Check sheet for the drawn part. Datum: minimum x, y, z corner. Units: mm. Coordinates: 2 decimals unless noted, no trailing zeros. Order: outer loops, then holes, each group sorted by start corner. A loop starts at its lowest first (then second) coordinate and runs counter-clockwise, first axis right, second up. Notation, with made-up numbers: (-20, 10.25) - (-7, 10.25) arc R16 ccw to (-7, 14.25) - close; hole circle Ø7 at (28.5, 34.5). An arc over 180 degrees is marked (long way). Put each result on its own line as item: value.
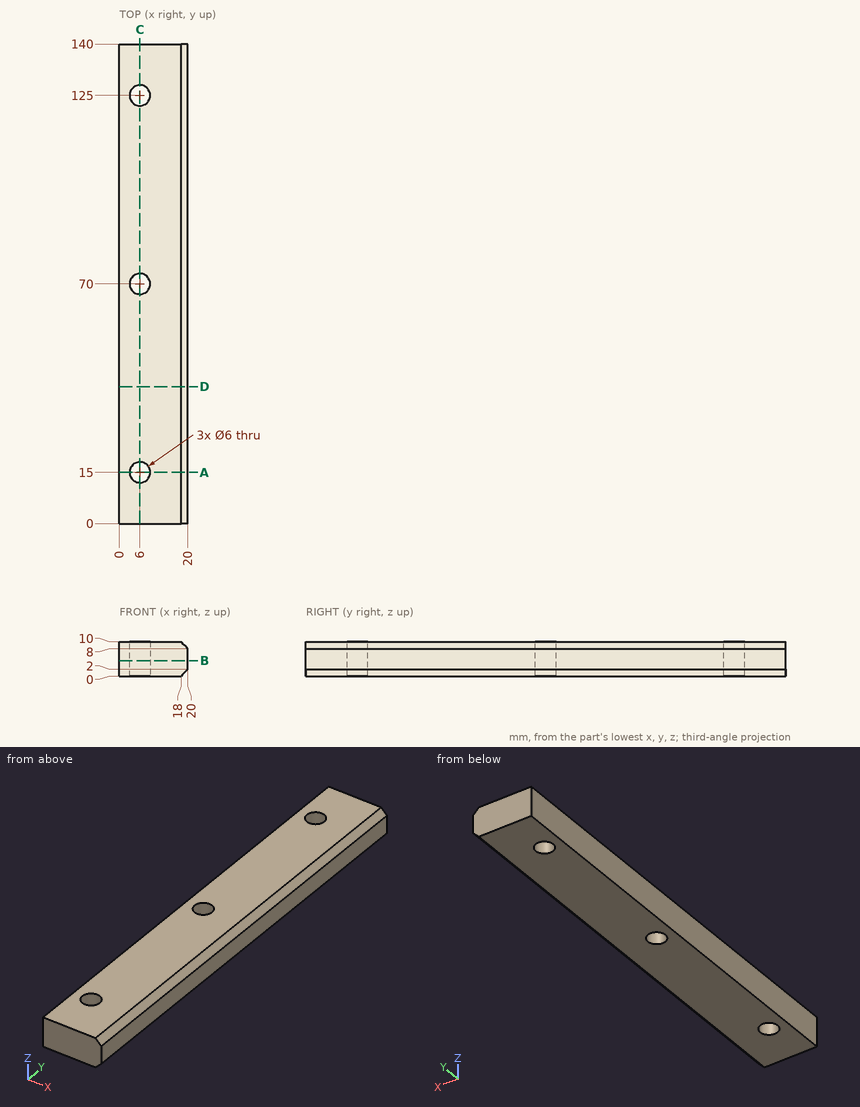
Q1. Thickness scan on L1, parallel to Y at x = 6, z = 7.5; L2, parallel to Y at x = 3.75, z = 3; L3, parallel to X at y = 81, z = 9.5. Record the ranges inside material, lowest first. Write a range as [from, to].
Answer block:
L1: y = [0, 12], [18, 67], [73, 122], [128, 140]
L2: y = [0, 13.02], [16.98, 68.02], [71.98, 123.02], [126.98, 140]
L3: x = [0, 18.5]
Q2. Section check C-C on x = 6. Record the boundary of the cut face in (y, z).
Answer block:
outline: (0, 0) - (12, 0) - (12, 10) - (0, 10) - close; (18, 0) - (67, 0) - (67, 10) - (18, 10) - close; (73, 0) - (122, 0) - (122, 10) - (73, 10) - close; (128, 0) - (140, 0) - (140, 10) - (128, 10) - close
Q3. Section check A-A on y = 15. Record the boundary of the cut face in (x, z), then the cut area to 3 significant figures.
Answer block:
outline: (0, 0) - (3, 0) - (3, 10) - (0, 10) - close; (9, 0) - (18, 0) - (20, 2) - (20, 8) - (18, 10) - (9, 10) - close
area: 136 mm^2
Q4. Section check B-B on z = 4.5. Record the boundary of the cut face in (x, y).
Answer block:
outline: (0, 0) - (20, 0) - (20, 140) - (0, 140) - close; hole circle Ø6 at (6, 15); hole circle Ø6 at (6, 70); hole circle Ø6 at (6, 125)
Q5. Section check D-D on y = 40. Record the boundary of the cut face in (x, z), then the cut area to 3 significant figures.
Answer block:
outline: (0, 0) - (18, 0) - (20, 2) - (20, 8) - (18, 10) - (0, 10) - close
area: 196 mm^2
Q6. Depth check by flat-ended pin: pin 1 Ø3.5 at (x, y) = (6, 70) entering from -Z. Enter the tip coordinate at first touch or a pass-through.
Answer block:
pin 1: passes through
